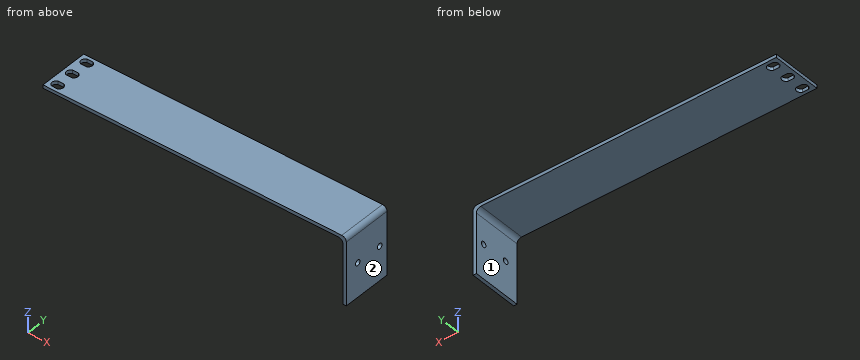
```python
from build123d import *

# Parameters (mm, degrees)
F0_W     = 270
F0_H     = 44.45
F1_DEPTH = 3
F3_DEPTH = 3
F2_W     = 3
F2_H     = 44.45
F4_DEPTH = 60
F5_R     = 2.5
F6_DEPTH = 3
F7_R     = 4
F8_R     = 4


# Not quite as in the source:
# - a feature names something its author has since deleted; it is built from what else it names


with BuildPart() as f1:
    # F0 (on Top) → F1 (new body)
    with BuildSketch(Plane.XY):
        with Locations((68.0511838198, -14.3298729897)):
            Rectangle(F0_W, F0_H)
    extrude(amount=F1_DEPTH)

    # F2 (on face) → F3 (cut)
    with BuildSketch(Plane.XY.offset(3)):
        with BuildLine():
            Line((-56.5113161802, -26.720496912), (-59.0113161802, -26.720496912))
            Line((-59.0113161802, -26.720496912), (-61.5113161802, -26.720496912))
            ThreePointArc((-61.5113161802, -26.720496912), (-64.0113244271, -30.220496912), (-61.5113161802, -33.720496912))
            Line((-61.5113161802, -33.720496912), (-59.0113161802, -33.720496912))
            Line((-59.0113161802, -33.720496912), (-56.5113161802, -33.720496912))
            ThreePointArc((-56.5113161802, -33.720496912), (-54.0113161802, -30.220496912), (-56.5113161802, -26.720496912))
        make_face()
        with BuildLine():
            Line((-61.5113161802, -17.845496912), (-59.0113161802, -17.845496912))
            Line((-59.0113161802, -17.845496912), (-56.5113161802, -17.845496912))
            ThreePointArc((-56.5113161802, -17.845496912), (-54.0113161802, -14.345496912), (-56.5113161802, -10.845496912))
            Line((-56.5113161802, -10.845496912), (-59.0113161802, -10.845496912))
            Line((-59.0113161802, -10.845496912), (-61.5113161802, -10.845496912))
            ThreePointArc((-61.5113161802, -10.845496912), (-64.0113244271, -14.345496912), (-61.5113161802, -17.845496912))
        make_face()
        with BuildLine():
            Line((-61.5113161802, -1.970496912), (-59.0113161802, -1.970496912))
            Line((-59.0113161802, -1.970496912), (-56.5113161802, -1.970496912))
            ThreePointArc((-56.5113161802, -1.970496912), (-54.0113161802, 1.529503088), (-56.5113161802, 5.029503088))
            Line((-56.5113161802, 5.029503088), (-59.0113161802, 5.029503088))
            Line((-59.0113161802, 5.029503088), (-61.5113161802, 5.029503088))
            ThreePointArc((-61.5113161802, 5.029503088), (-64.0113244271, 1.529503088), (-61.5113161802, -1.970496912))
        make_face()
    extrude(amount=-F3_DEPTH, mode=Mode.SUBTRACT)

    # F2 (on face) → F4 (join)
    with BuildSketch(Plane.XY.offset(3)):
        with Locations((201.5511838198, -14.3298729897)):
            Rectangle(F2_W, F2_H)
    extrude(amount=-F4_DEPTH)

    # F5 (on face) → F6 (cut)
    with BuildSketch(Plane.YZ.offset(203.0511838198)):
        with Locations((-24.0548729897, -26.75)):
            Circle(F5_R)
        with Locations((-0.0548729897, -26.75)):
            Circle(F5_R)
    extrude(amount=-F6_DEPTH, mode=Mode.SUBTRACT)

    # F7
    f7_edges = [f1.edges().sort_by_distance(p)[0] for p in [
        (200.051184, -14.329873, 0),
    ]]
    fillet(f7_edges, radius=F7_R)

    # F8
    f8_edges = [f1.edges().sort_by_distance(p)[0] for p in [
        (203.051184, -14.329873, 3),
    ]]
    fillet(f8_edges, radius=F8_R)


solid = f1.part
```
Work out the finished part from the listing and answer in its coordinate system (mm). Face numbers are marked on the shaded views. A direction names the side the tool comes from. Coordinates: 2 decimals unless noted, no trailing zeros. Order: outer loops, then holes, each group sorted by start corner. A loop starts at its lowest first (then second) coordinate and runs counter-clockwise, first axis right, second up. Notation, with made-up numbers: M 20.5,41.5 L 58.5,41.5 A21 ccw 58.5,55.5 Z; hole C -2.5,-6.75 d9. An arc over 180 degrees is marked long. Use CSV: the item, a comma, the result in double quotes.
1) Section A-A on z = -26.75 is taken. Write down the section's boundary in (x, y), plus the area to 3 significant figures.
Worked out:
outline,"M 200.05,-36.55 L 203.05,-36.55 L 203.05,-26.55 L 200.05,-26.55 Z; M 200.05,-21.55 L 203.05,-21.55 L 203.05,-2.55 L 200.05,-2.55 Z; M 200.05,2.45 L 203.05,2.45 L 203.05,7.9 L 200.05,7.9 Z"
area,"103 mm^2"
2) For the marked faces 1 and 2, determine the directions among +Z, -Z, +X, -X, +Y, -Y from which every point of the face is accessible in a straight line to the end or side of a thin tool.
Worked out:
face 1,"-Z, -X, +Y, -Y"
face 2,"+Z, -Z, +X, +Y, -Y"
3) Section C-C on x = -2 is taken. Write down the section's boundary in (y, z), plus the area to 3 significant figures.
Worked out:
outline,"M -36.55,0 L 7.9,0 L 7.9,3 L -36.55,3 Z"
area,"133 mm^2"
4) Consider line 1 (Y direction, x = 202, z = -26); line 2 (Z direction, x = 158.5, y = -18); line 3 (X direction, y = -32, z = -13). Determine where each line is inside the solid, lowest interval first. Write a range as [from, to].
Worked out:
line 1,"y = [-36.55, -26.44], [-21.67, -2.44], [2.33, 7.9]"
line 2,"z = [0, 3]"
line 3,"x = [200.05, 203.05]"
5) Section B-B on y = -29 is taken. Write down the section's boundary in (x, z), plus the area to 3 significant figures.
Worked out:
outline,"M -66.95,0 L -63.8,0 L -63.8,3 L -66.95,3 Z; M -54.22,0 L 196.05,0 A4 cw 200.05,-4 L 200.05,-57 L 203.05,-57 L 203.05,-1 A4 ccw 199.05,3 L -54.22,3 Z"
area,"952 mm^2"
6) Flat-ended cylindrical pins translate along their axes: pin 1 Ø10 at (y, z) = (-9.5, -4) entering from -X; pin 2 Ø1.5 at (y, z) = (-16.5, -13) entering from -X; pin 3 Ø3 at (x, y) = (-18.5, -14) entering from -Z. Find the tip coordinate at first contact, or state that the pin passes through.
Worked out:
pin 1,"stops at x = -66.95"
pin 2,"stops at x = 200.05"
pin 3,"stops at z = 0"
